Autodesk Inventor part; units mm, degrees
ref_plane "Work Plane1" through (29, 0, 0) normal (0, -1, 0) x (1, 0, 0)
ref_plane "YZ Plane" through (0, 0, 0) normal (1, 0, 0) x (0, 1, 0)
ref_plane "XZ Plane" through (0, 0, 0) normal (0, 1, 0) x (-1, 0, 0)
sketch "Эскиз1" plane through (0, 0, 0) normal (0, 0, 1) x (1, 0, 0)
  line L0 (-1, 0) -> (25, 0)
  line L1 (25, 0) -> (25, 2)
  line L2 (25, 2) -> (11, 2)
  line L3 (11, 2) -> (10.5705, 1.7853)
  line L4 (10.5705, 1.7853) -> (0, 1.7853)
  line L5 (0, 1.7853) -> (0, 3.5)
  line L6 (0, 3.5) -> (-4, 3.5)
  line L7 (-4, 3.5) -> (-4, 1.7321)
  line L8 (-4, 1.7321) -> (-2, 1.7321)
  line L9 (-2, 1.7321) -> (-1, 0)
  line L10 (-9.8, 0) -> (30.8, 0)
  line L11 (0, -0.7) -> (0, 4.2)
  line L12 (11, 2) -> (0, 2) construction
  dimension "d1" = 14
  dimension "d2" = 0.4295
  dimension "d3" = 4
  dimension "d4" = 2
  dimension "d5" = 60
  dimension "d6" = 4
  dimension "d7" = 3.5705
  dimension "d8" = 3.4641
  dimension "d9" = 7
  dimension "d26" = 25
revolve "Базовый элемент" add sketch "Эскиз1" angle 360 about axis through (-1, 0, 0) along (1, 0, 0)
sketch "Эскиз2" plane through (-4, 0, 0) normal (-1, 0, 0) x (0, 0, 1)
  circle A0 centre (0, 0) radius 1.7321
  line L0 (0, -4.9) -> (0, 4.9)
  line L1 (-4.9, 0) -> (4.9, 0)
  line L2 (1.7321, 0) -> (0.866, -1.5)
  line L3 (0.866, -1.5) -> (-0.866, -1.5)
  line L4 (-0.866, -1.5) -> (-1.7321, 0)
  line L5 (-1.7321, 0) -> (-0.866, 1.5)
  line L6 (-0.866, 1.5) -> (0.866, 1.5)
  line L7 (0.866, 1.5) -> (1.7321, 0)
extrude "Паз" add sketch "Эскиз2" against normal up to next contours L7 A0 | A0 L2 | L6 L0 A0 | A0 L0 L3 | L0 L6 A0 | A0 L3 L0 | L4 A0 | A0 L5
fillet "Сопряжение1" radius 0.4 1 edges at (-4, -3.5, 0)
thread "Резьба"
chamfer "Фаска1" distance 0.4294 distance2 0.4294 1 edges at (25, -2, 0) measured on face at (25, 0.6473, 0.1595)
ref_plane "Work Plane1" through (29, 0, 0) normal (0, -1, 0) x (1, 0, 0)
fillet "Fillet2" radius 0.1 1 edges at (0, -1.7853, 0)
equation "\"d1\" = GEL"
equation "\"d3\" = KOH"
equation "\"d4\" = INTI"
equation "\"d6\" = GD"
equation "\"d7\" = BDM"
equation "\"d8\" = 1.1547 * SW"
equation "\"d9\" = KOD"
equation "\"d26\" = NLG"
equation "\"d30\" = R"
equation "\"d17\" = RR"
equation "\"d13\" = GEL"
equation "\"d15\" = -0.5 * SPD + 0.5 * GD"
equation "\"d16\" = GUL"
equation "\"GD\" = NND"
equation "\"NLG\" = 25"
equation "\"GEL\" = 14"
equation "\"KOD\" = 7"
equation "\"KOH\" = NND"
equation "\"INTI\" = 2"
equation "\"GAL\" = 0.61345 * PTC"
equation "\"GUL\" = 0.61345 * PTC"
equation "\"BDM\" = 3.5705"
equation "\"SW\" = 3"
equation "\"RR\" = 0.4"
equation "\"SPD\" = NND - 1.2269 * PTC"
equation "\"R\" = 0.1"
equation "\"PHH\" = 0.4"
equation "\"GD1\" = THREADDIA - 1.2269 * PTC"
equation "\"THREADDIA\" = 4"
equation "\"FAWI\" = 45deg"
equation "\"PTC\" = 0.7"
equation "\"NND\" = 4"
equation "\"TOA\" = 30deg"
equation "\"E0\" = 1.155 * SW"
properties part number "CSN 02 1143 - M4 x 25" material "Сталь, мягкая"
Could you check a few things on this model? Use its own coordinates, in mm. A direction names the side the tool comes from. Give positions to 0.01 mm unless a question says otherwise; leave off trailing zeros. Write each loop counter-clockwise with the first axis right and the second up, starting at its lowest first coordinate (ties: lowest second). Pieces come first, ordered by that corner, then holes. Notation, with made-up numbers: (89, 8) -> (124, 8) arc R33 ccw to (124, 45) -> close; hole circle Ø8 at (19, -5.75). An arc over 180 degrees is marked (long way). Answer as CSV lines item,"result". Start each with the question number.
(1) Please list where these lines run through material, in increasing order: line 1 (X direction, y = 2, z = 1); line 2 (X direction, y = 1.75, z = 0.75); line 3 (Y direction, x = 21.75, z = 1).
(2) Which directions (+Z, -Z, +X, -X, +Y, -Y) give clear straight access to the entire face, cutting with the end or side of a thin tool? Please do faces 1 (the face through (-1.825, 3.233, 1.341)), 2 (the face through (5.262, -0.387, 1.743)), 3 (the face through (-2.948, 0.74, -1.305)).
(3) If we section it at C-C, the plane x = 6: Write out the boundary of the cut face in (y, z).
(4) If we section it at A-A, the plane x = 14.25: Write out the boundary of the cut face in (y, z).
(5) If we mould it in two halves opening along Y, with no side actions, what happens to faces 4 (the face through (-4, -1.3, 1.3)), 5 (the face through (-2.948, -0.74, 1.305)), 6 (the face through (18, 0, 2))? For each: +Y half, -Y half, draft (parallel to the pull), parting line (faces both ways), or undercut.
(6) I'm going to push flat-ended pins straight in: pin 1 Ø1.5 at (x, z) = (9, 1.5) entering from +Y; pin 2 Ø1.5 at (x, y) = (21.5, 2.5) entering from -Z. Where does each tip first touch, or does it pass through?
(7) If we section it at B-B, the plane x = -1.25: Write out the boundary of the cut face in (y, z).
Answer list:
1,line 1,"-4 to 0"
1,line 2,"-4 to 0, 10.81 to 24.67"
1,line 3,"-1.73 to 1.73"
2,face 1,"+X, -X"
2,face 2,"none"
2,face 3,"-X"
3,outline,"circle Ø3.57 at (0, 0)"
4,outline,"circle Ø4 at (0, 0)"
5,face 4,"draft"
5,face 5,"undercut"
5,face 6,"parting line"
6,pin 1,"y = 1.62"
6,pin 2,"z = -0.97"
7,outline,"circle Ø7 at (0, 0); hole circle Ø0.87 at (0, 0)"
